The listing builds one solid part. Answer for the finished solid, in the listing's coordinates (mm). A direction names the side the tool comes from. Give positions to 0.01 mm unless a question says otherwise; leave off trailing zeros. Order: outer loops, then holes, each group sorted by start corner. A loop starts at its lowest first (then second) coordinate and runs counter-clockwise, first axis right, second up. Notation, with made-up numbers: (-13, 83) - (-4, 83) arc R32 ccw to (-4, 116) - close; hole circle Ø11 at (33, 80). An arc over 180 degrees is marked (long way). Answer in a Markdown table with one row per item.
from build123d import *

# Parameters (mm, degrees)
SCHIZZO1_W                   = 380
SCHIZZO1_H                   = 100
ESTRUSIONE_ESTRUSIONE1_DEPTH = 10
SCHIZZO2_R                   = 54
TAGLIO_ESTRUSIONE1_DEPTH     = 2
SCHIZZO3_R                   = 2.75
TAGLIO_ESTRUSIONE2_DEPTH     = 197.631635298
RIPETIZIONECIRCOLARE1_COUNT  = 8
SCHIZZO4_R                   = 34
TAGLIO_ESTRUSIONE3_DEPTH     = 197.631635298
SCHIZZO5_R                   = 3.4
TAGLIO_ESTRUSIONE4_DEPTH     = 197.723155729


with BuildPart() as part:
    # Schizzo1 → Estrusione-Estrusione1 (new body)
    with BuildSketch(Plane.XY):
        Rectangle(SCHIZZO1_W, SCHIZZO1_H)
    extrude(amount=ESTRUSIONE_ESTRUSIONE1_DEPTH)

    # Schizzo2 → Taglio-Estrusione1 (cut)
    with BuildSketch(Plane.XY.offset(10)):
        Circle(SCHIZZO2_R)
    extrude(amount=-TAGLIO_ESTRUSIONE1_DEPTH, mode=Mode.SUBTRACT)

    # Schizzo3 → Taglio-Estrusione2 (cut, through all)
    with BuildSketch(Plane.XY.offset(8)):
        with Locations((-44.346217561, -18.368804754)):
            Circle(SCHIZZO3_R)
    taglio_estrusione2 = extrude(amount=-TAGLIO_ESTRUSIONE2_DEPTH, mode=Mode.SUBTRACT)

    # RipetizioneCircolare1: Taglio-Estrusione2 ×8 about axis
    ripetizionecircolare1_axis = Axis((0, 0, 0), (0, 0, 1))
    for i in range(1, RIPETIZIONECIRCOLARE1_COUNT):
        add(taglio_estrusione2.rotate(ripetizionecircolare1_axis, i * 360 / RIPETIZIONECIRCOLARE1_COUNT), mode=Mode.SUBTRACT)

    # Schizzo4 → Taglio-Estrusione3 (cut, through all)
    with BuildSketch(Plane.XY.offset(8)):
        Circle(SCHIZZO4_R)
    extrude(amount=-TAGLIO_ESTRUSIONE3_DEPTH, mode=Mode.SUBTRACT)

    # Schizzo5 → Taglio-Estrusione4 (cut, through all)
    with BuildSketch(Plane.XY.offset(10)):
        with Locations((-150, 0)):
            Circle(SCHIZZO5_R)
    extrude(amount=-TAGLIO_ESTRUSIONE4_DEPTH, mode=Mode.SUBTRACT)


solid = part.part
Item 1: Which of the six approach directions +Z, -Z, +X, -X, +Y, -Y give full straight-line access (tool end or side, diameter ignored) to faces 1 (the face through (190, -1, 5)), 2 (the face through (-53.993, 0.895, 9.014))?
Answer block:
| item | result |
|---|---|
| face 1 | +Z, -Z, +X, +Y, -Y |
| face 2 | +Z |
Item 2: Consider line 1 (Y direction, x = 0, z = 3); line 2 (Y direction, x = -150, z = 3.25); line 3 (X direction, y = -1.5, z = 1.5). Determine where each line is inside the solid, lowest interval first.
Answer block:
| item | result |
|---|---|
| line 1 | -50 to -34, 34 to 50 |
| line 2 | -50 to -3.4, 3.4 to 50 |
| line 3 | -190 to -153.05, -146.95 to -33.97, 33.97 to 190 |
Item 3: Each of these flat-tipped pins is pushed along its axis until it touches: P1, Ø4.5, axis at x = 18.37, y = -44.35, coming from the -Z side; P2, Ø7, axis at x = -44.35, y = -18.37, coming from the +Z side. Where does it stop, or does it pass through?
Answer block:
| item | result |
|---|---|
| P1 | through |
| P2 | z = 8 |
Item 4: Determine the mould class of faces 3 (the face through (-3, -50, 5)), 4 (the face through (53.993, -0.895, 9.014)), 5 (the face through (-153.4, 0.1, 5.1)), 6 (the face through (-125, 1, 10)) for opening direction Y: pulls with the +Y half, pulls with the -Y half, needs draft (parallel to the pull), parting line crosses it, or undercut.
Answer block:
| item | result |
|---|---|
| face 3 | pulls with the -Y half |
| face 4 | undercut |
| face 5 | undercut |
| face 6 | needs draft |
Item 5: Find section B-B on y = 0. Write down the section's boundary in (x, z), then the cut area to 3 significant figures.
Answer block:
| item | result |
|---|---|
| outline | (-190, 0) - (-153.4, 0) - (-153.4, 10) - (-190, 10) - close; (-146.6, 0) - (-34, 0) - (-34, 8) - (-54, 8) - (-54, 10) - (-146.6, 10) - close; (34, 0) - (190, 0) - (190, 10) - (54, 10) - (54, 8) - (34, 8) - close |
| area | 2,970 mm² |
Item 6: Find section C-C on y = -25.5. Write down the section's boundary in (x, z).
Answer block:
| item | result |
|---|---|
| outline | (-190, 0) - (-22.49, 0) - (-22.49, 8) - (-47.6, 8) - (-47.6, 10) - (-190, 10) - close; (22.49, 0) - (190, 0) - (190, 10) - (47.6, 10) - (47.6, 8) - (22.49, 8) - close |
Item 7: Find section D-D on z = 1.5. Count the separate pieces of the cut face and the enclosed holes in it, then the cut area to 3 significant figures.
Answer block:
| item | result |
|---|---|
| separate pieces | 1 |
| enclosed holes | 10 |
| area | 34,100 mm² |
Item 8: Find section A-A on x = 0. Write down the section's boundary in (y, z), then the cut area to 3 significant figures.
Answer block:
| item | result |
|---|---|
| outline | (-50, 0) - (-34, 0) - (-34, 8) - (-50, 8) - close; (34, 0) - (50, 0) - (50, 8) - (34, 8) - close |
| area | 256 mm² |
